Verification items for the finished model (mm, model axes). A direction names the side the tool comes from. Give positions to 0.01 mm unless a question says otherwise; leave off trailing zeros. Order: outer loops, then holes, each group sorted by start corner. A loop starts at its lowest first (then second) coordinate and runs counter-clockwise, first axis right, second up. Notation, with made-up numbers: (2, 88) - (7, 88) arc R22 ccw to (7, 108) - close; hole circle Ø5 at (68, 52.5). An arc over 180 degrees is marked (long way). Answer as a JSON object with one key per item and string values. Group by question number.
(1) Section check A-A (x = 0). Record the boundary of the cut face in (y, z) (3 decimals), then the cut area to 3 significant figures.
(2) Section check D-D (z = -9). Record the boundary of the cut face in (x, y) (3 decimals).
(3) Section check B-B (z = 0). Count the separate pieces of the cut face and the enclosed holes in it, then the cut area to 3 significant figures.
(4) Thickness scan on line 1 (X direction, y = 29.5, z = 10) (3 decimals); line 2 (Y direction, x = -39, z = -3) (3 decimals); line 3 (X direction, y = 4, z = -15.5) (3 decimals). Record the ranges inside material, lowest first.
(5) Mould release check, pull along X, two halves, no side actions. Record for faces 5 (the face through (0.089, 40.041, -24.756)), 6 (the face through (48.7, 3.175, 2.9)), 7 (the face through (57.785, 2, 0)): +X half, -X half, draft (parallel to the pull), parting line (faces both ways), or undercut.
(6) Section check C-C (y = 8.5). Record the boundary of the cut face in (x, z) (3 decimals).
(7) Depth check by flat-ended pin: pin 1 Ø24 at (x, y) = (-7, 25) entering from +Z (3 decimals); pin 2 Ø0.6 at (y, z) = (45, -24.5) entering from +X (3 decimals); pin 3 Ø1.9 at (x, z) = (38, 1.5) entering from +Y (3 decimals). Enter the tip coordinate at first touch or a pass-through.
(8) Access from +Z, -Z, +X, -X, +Y, -Y to the whole of each face (thin tool, end or side, straight path). Record for faces 1 (the face through (51, 2, -6.35)), 2 (the face through (43.52, 15.14, 23.15)), 3 (the face through (-39, 12.7, 2)), 4 (the face through (35.56, 5, 2)).
Autodesk Inventor part; units mm, degrees
ref_plane "YZ Plane" through (0, 0, 0) normal (1, 0, 0) x (0, 1, 0)
ref_plane "XZ Plane" through (0, 0, 0) normal (0, 1, 0) x (-1, 0, 0)
ref_plane "XY Plane" through (0, 0, 0) normal (0, 0, 1) x (1, 0, 0)
sketch "Sketch1" plane through (0, 0, 0) normal (0, 1, 0) x (-1, 0, 0)
  line L0 (45.085, 25.4) -> (-45.085, 25.4)
  line L1 (-45.085, 25.4) -> (-45.085, -25.4)
  line L2 (-45.085, -25.4) -> (45.085, -25.4)
  line L3 (45.085, -25.4) -> (45.085, 25.4)
  point P0 (0, 0)
  dimension "d0" = 90.17
  dimension "d1" = 45.085
  dimension "d2" = 50.8
  dimension "d3" = 25.4
extrude "Extrusion1" add sketch "Sketch1" along normal blind 50.8
sketch "Sketch2" plane through (0, 0, 0) normal (0, 1, 0) x (-1, 0, 0)
  line L0 (45.085, -25.4) -> (45.085, 25.4)
  line L1 (45.085, 6.35) -> (57.785, 6.35)
  line L2 (57.785, 6.35) -> (57.785, -6.35)
  line L3 (57.785, -6.35) -> (45.085, -6.35)
  line L4 (45.085, -6.35) -> (45.085, 6.35)
  line L5 (-45.085, 25.4) -> (-45.085, -25.4)
  line L6 (-45.085, -6.35) -> (-57.785, -6.35)
  line L7 (-57.785, -6.35) -> (-57.785, 6.35)
  line L8 (-57.785, 6.35) -> (-45.085, 6.35)
  line L9 (-45.085, 6.35) -> (-45.085, -6.35)
  circle A0 centre (51.435, 0) radius 3.81
  circle A1 centre (-51.435, 0) radius 3.81
  line L10 (51.435, 0) -> (51.435, -6.35) construction
  point P0 (0, 0)
  point P1 (-45.085, 6.35)
  point P2 (45.085, -6.35)
  dimension "d6" = 12.7
  dimension "d7" = 12.7
  dimension "d8" = 6.35
  dimension "d9" = 7.62
  dimension "d34" = 6.35
  dimension "d35" = 6.35
  dimension "d37" = 6.35
extrude "Extrusion2" add sketch "Sketch2" along normal blind 3.175
sketch "Sketch4" plane through (-45.085, 0, 25.4) normal (0, 0, 1) x (1, 0, 0)
  line L0 (9.525, 3.175) -> (80.645, 3.175)
  line L1 (90.17, 0) -> (90.17, 50.8)
  line L2 (0, 50.8) -> (90.17, 50.8)
  line L3 (0, 0) -> (90.17, 0)
  line L4 (3.175, 40.8121) -> (3.175, 50.8)
  line L5 (90.17, 50.8) -> (0, 50.8)
  circle A0 centre (13.335, 40.8121) radius 2.5681 construction
  circle A1 centre (29.21, 40.8121) radius 2.5681 construction
  circle A2 centre (45.085, 40.8121) radius 2.6318 construction
  circle A3 centre (60.96, 40.8121) radius 2.9599 construction
  circle A4 centre (76.835, 40.8121) radius 2.9663 construction
  line L6 (3.175, 40.8121) -> (13.335, 40.8121) construction
  line L7 (13.335, 40.8121) -> (29.21, 40.8121) construction
  line L8 (29.21, 40.8121) -> (45.085, 40.8121) construction
  line L9 (45.085, 40.8121) -> (60.96, 40.8121) construction
  line L10 (60.96, 40.8121) -> (76.835, 40.8121) construction
  line L11 (76.835, 40.8121) -> (86.995, 40.8121) construction
  line L12 (3.175, 6.35) -> (9.525, 12.7)
  line L13 (9.525, 12.7) -> (3.175, 12.7)
  line L14 (3.175, 22.225) -> (9.525, 28.575)
  line L15 (9.525, 28.575) -> (3.175, 28.575)
  line L16 (45.085, 3.175) -> (45.085, 50.8) construction
  line L17 (3.175, 22.225) -> (3.175, 12.7)
  line L18 (0, 0) -> (0, 50.8)
  line L19 (90.17, 0) -> (0, 0)
  line L20 (3.175, 6.35) -> (9.525, 6.35)
  line L21 (9.525, 6.35) -> (9.525, 3.175)
  line L22 (86.995, 6.35) -> (80.645, 6.35)
  line L23 (80.645, 6.35) -> (80.645, 3.175)
  line L24 (3.175, 28.575) -> (3.175, 40.8121)
  line L25 (86.995, 12.7) -> (86.995, 6.35)
  line L26 (86.995, 6.35) -> (80.645, 12.7)
  line L27 (80.645, 12.7) -> (86.995, 12.7)
  line L28 (86.995, 22.225) -> (80.645, 28.575)
  line L29 (80.645, 28.575) -> (86.995, 28.575)
  line L30 (86.995, 22.225) -> (86.995, 12.7)
  line L31 (86.995, 28.575) -> (86.995, 40.8121)
  line L32 (86.995, 40.8121) -> (86.995, 50.8)
  line L33 (90.17, 0) -> (90.17, 50.8)
  point P0 (45.085, 0)
  point P1 (3.175, 6.35)
  dimension "d15" = 3.175
  dimension "d19" = 15.875
  dimension "d22" = 6.35
  dimension "d23" = 9.525
  dimension "d25" = 6.35
  dimension "d26" = 25.4
  dimension "d39" = 6.35
  dimension "d40" = 6.35
  dimension "d41" = 3.175
  dimension "d42" = 3.175
extrude "Extrusion3" cut sketch "Sketch4" against normal blind 47.625 contours L21 L20 L12 L13 L17 L14 L15 L24 L4 L2 L32 L31 L29 L28 L30 L27 L26 L22 L23 L0
sketch "Sketch5" plane through (-45.085, 0, -22.225) normal (0, 0, 1) x (1, 0, 0)
  line L0 (3.175, 12.065) -> (3.175, 22.225)
  line L1 (19.7358, 22.225) -> (32.4104, 22.225) construction
  line L2 (32.4104, 22.225) -> (45.085, 22.225) construction
  line L3 (45.085, 22.225) -> (57.7596, 22.225) construction
  line L4 (57.7596, 22.225) -> (70.4342, 22.225) construction
  line L5 (86.995, 22.225) -> (86.995, 12.065)
  circle A0 centre (19.7358, 22.225) radius 3.81
  circle A1 centre (32.4104, 22.225) radius 3.81
  circle A2 centre (45.085, 22.225) radius 3.81
  circle A3 centre (57.7596, 22.225) radius 3.81
  circle A4 centre (70.4342, 22.225) radius 3.81
  line L6 (19.7358, 22.225) -> (3.175, 22.225) construction
  line L7 (70.4342, 22.225) -> (86.995, 22.225) construction
  line L8 (80.645, 3.175) -> (9.525, 3.175)
  line L9 (0, 0) -> (90.17, 0)
  point P0 (45.085, 0)
  point P1 (86.995, 3.175)
  point P2 (3.175, 3.175)
  dimension "d29" = 12.6746
  dimension "d30" = 7.62
  dimension "d38" = 22.225
extrude "Extrusion4" cut sketch "Sketch5" against normal blind 47.625
sketch "Sketch7" plane through (0, 0, 0) normal (1, 0, 0) x (0, 1, 0)
  line L0 (0, -25.4) -> (50.8, -25.4)
  line L1 (50.8, -25.4) -> (47.625, -25.4)
  line L2 (47.625, -25.4) -> (42.545, -24.13)
  line L3 (42.545, -24.13) -> (37.465, -25.4)
  line L4 (37.465, -25.4) -> (47.625, -25.4)
  line L5 (50.8, 25.4) -> (50.8, -25.4)
  point P0 (0, 0)
  point P1 (37.465, -25.4)
  dimension "d43" = 3.175
  dimension "d44" = 1.27
  dimension "d45" = 10.16
extrude "Extrusion5" cut sketch "Sketch7" against normal mid plane 12.7
sketch "Sketch8" plane through (45.085, 0, -25.4) normal (1, 0, 0) x (0, 0, -1)
  line L0 (-50.8, 12.7) -> (-50.8, 12.8905) construction
  line L1 (-50.8, 0) -> (-50.8, 50.8) construction
  line L2 (-50.8, 12.8905) -> (-46.228, 17.4625)
  line L3 (-46.228, 17.4625) -> (-50.8, 22.0345)
  line L4 (-50.8, 22.0345) -> (-50.8, 22.225) construction
  line L5 (-50.8, 22.225) -> (-3.175, 22.225) construction
  line L6 (-50.8, 22.225) -> (-46.228, 22.225) construction
  line L7 (-46.228, 22.225) -> (-46.228, 17.4625) construction
  line L8 (-46.228, 17.4625) -> (-46.228, 12.7) construction
  line L9 (-50.8, 12.7) -> (-3.175, 12.7) construction
  line L10 (-46.228, 12.7) -> (-50.8, 12.7) construction
  line L11 (-50.8, 22.0345) -> (-50.8, 12.8905)
  point P0 (-25.4, 0)
  dimension "d48" = 45
  dimension "d49" = 45
  dimension "d50" = 4.572
extrude "Extrusion6" cut sketch "Sketch8" against normal blind 25.4
equation "\"d34\" = 0.5 * d6"
equation "\"d35\" = d34"
equation "\"d37\" = d8"
equation "\"d15\" = d12"
equation "\"d42\" = d41"
properties part number "PCB_Case02"
Solutions:
{
 "1": {"outline": "(0, -25.4) - (18.415, -25.4) - (18.415, -22.225) - (3.175, -22.225) - (3.175, 25.4) - (0, 25.4) - close; (26.035, -25.4) - (37.465, -25.4) - (42.545, -24.13) - (47.625, -25.4) - (50.8, -25.4) - (50.8, -22.225) - (26.035, -22.225) - close", "area": "282 mm2"},
 "2": {"outline": "(-45.085, 0) - (45.085, 0) - (45.085, 50.8) - (41.91, 50.8) - (41.91, 28.575) - (35.56, 28.575) - (41.91, 22.225) - (41.91, 12.7) - (35.56, 12.7) - (41.91, 6.35) - (35.56, 6.35) - (35.56, 3.175) - (-35.56, 3.175) - (-35.56, 6.35) - (-41.91, 6.35) - (-35.56, 12.7) - (-41.91, 12.7) - (-41.91, 22.225) - (-35.56, 28.575) - (-41.91, 28.575) - (-41.91, 50.8) - (-45.085, 50.8) - close"},
 "3": {"separate pieces": "3", "enclosed holes": "0", "area": "742 mm2"},
 "4": {"line 1": "x = -45.085 to -41.91, 41.91 to 45.085", "line 2": "y = 0 to 6.35, 9.26 to 12.7, 25.135 to 28.575", "line 3": "x = -45.085 to -35.56, 35.56 to 45.085"},
 "5": {"face 5": "undercut", "face 6": "draft", "face 7": "+X half"},
 "6": {"outline": "(-45.085, -25.4) - (45.085, -25.4) - (45.085, 25.4) - (39.76, 25.4) - (39.76, -22.225) - (-39.76, -22.225) - (-39.76, 25.4) - (-45.085, 25.4) - close"},
 "7": {"pin 1": "stops at z = -22.225", "pin 2": "stops at x = 45.085", "pin 3": "stops at y = 28.575"},
 "8": {"face 1": "-Z, +X, +Y, -Y", "face 2": "+Z, +X", "face 3": "+Z", "face 4": "+Z, +Y"}
}
